from build123d import *

# Parameters (mm, degrees)
SKETCH1_R                    = 203.2
BOSS_EXTRUDE1_DEPTH          = 6.35
F_0_257_DIAMETER_HOLE1_D     = 6.5278
CIRPATTERN1_COUNT            = 36
F_1_2_0_5_DIAMETER_HOLE1_D   = 12.7
F_3_8_0_375_DIAMETER_HOLE1_D = 9.525
CIRPATTERN2_COUNT            = 4
F_3_8_0_375_DIAMETER_HOLE2_D = 9.525
LPATTERN1_COUNT              = 2
LPATTERN1_PITCH              = 254
LPATTERN1_COUNT_DIR2         = 2
LPATTERN1_PITCH_DIR2         = 76.2


with BuildPart() as part:
    # Sketch1 → Boss-Extrude1 (new body)
    with BuildSketch(Plane(origin=(0, 0, 0), x_dir=(0, 0, -1), z_dir=(1, 0, 0))):
        Circle(SKETCH1_R)
    extrude(amount=BOSS_EXTRUDE1_DEPTH)

    # F (0.257) Diameter Hole1 (through all)
    with Locations(Plane(origin=(6.35, 0, 0), x_dir=(0, 0, -1), z_dir=(1, 0, 0))):
        with Locations((-196.85, 0)):
            f_0_257_diameter_hole1 = Hole(F_0_257_DIAMETER_HOLE1_D / 2)

    # CirPattern1: F (0.257) Diameter Hole1 ×36 about axis
    cirpattern1_axis = Axis((0, 0, 0), (-1, 0, 0))
    for i in range(1, CIRPATTERN1_COUNT):
        add(f_0_257_diameter_hole1.rotate(cirpattern1_axis, i * 360 / CIRPATTERN1_COUNT), mode=Mode.SUBTRACT)

    # 1/2 (0.5) Diameter Hole1 (through all)
    with Locations(Plane(origin=(6.35, 0, 0), x_dir=(0, 0, -1), z_dir=(1, 0, 0))):
        with Locations((0, 0)):
            Hole(F_1_2_0_5_DIAMETER_HOLE1_D / 2)

    # 3/8 (0.375) Diameter Hole1 (through all)
    with Locations(Plane(origin=(6.35, 0, 0), x_dir=(0, 0, -1), z_dir=(1, 0, 0))):
        with Locations((0, -76.2)):
            f_3_8_0_375_diameter_hole1 = Hole(F_3_8_0_375_DIAMETER_HOLE1_D / 2)

    # CirPattern2: 3/8 (0.375) Diameter Hole1 ×4 about axis
    cirpattern2_axis = Axis((0, 0, 0), (-1, 0, 0))
    for i in range(1, CIRPATTERN2_COUNT):
        add(f_3_8_0_375_diameter_hole1.rotate(cirpattern2_axis, i * 360 / CIRPATTERN2_COUNT), mode=Mode.SUBTRACT)

    # 3/8 (0.375) Diameter Hole2 (through all)
    with Locations(Plane(origin=(6.35, 0, 0), x_dir=(0, 0, -1), z_dir=(1, 0, 0))):
        with Locations((-127, -38.1)):
            f_3_8_0_375_diameter_hole2 = Hole(F_3_8_0_375_DIAMETER_HOLE2_D / 2)

    # LPattern1: 3_8 _0.375_ Diameter Hole2 2 × 2
    with Locations(*[(0, j * LPATTERN1_PITCH_DIR2, -i * LPATTERN1_PITCH) for i in range(LPATTERN1_COUNT) for j in range(LPATTERN1_COUNT_DIR2) if (i, j) != (0, 0)]):
        add(f_3_8_0_375_diameter_hole2, mode=Mode.SUBTRACT)


solid = part.part
Work out the finished part from the listing and answer in its coordinate system (mm). Give positions to 0.01 mm unless a question says otherwise; leave off trailing zeros. Loops run counter-clockwise (first coordinate to the right, second up) from the corner with the lowest first, then second, coordinate; pieces in that order, holes last. Notation, with made-up numbers: (-8, -6) - (24, -6) arc R19 cw to (24, 24) - close; hole circle Ø10 at (-28.5, 38). An arc over 180 degrees is marked (long way). Answer in a Markdown table with one row per item.
(1) A flat-ended cylindrical pin translates along its axis: pin 1 Ø4 at (y, z) = (-170.48, -98.43) entering from -X. Find the tip coordinate at first contact, or state that the pin passes through.
Results list:
| item | result |
|---|---|
| pin 1 | passes through |
(2) Consider L1, parallel to Y at x = 4.5, z = -66; L2, parallel to Z at x = 3.5, y = 67.5; L3, parallel to Y at x = 2.5, z = -1.5. Determine where each line is inside the solid, lowest interval first. Write a range as [from, to].
Results list:
| item | result |
|---|---|
| L1 | y = [-192.18, -187.96], [-182, 182], [187.96, 192.18] |
| L2 | z = [-191.66, -188.24], [-181.72, 181.72], [188.24, 191.66] |
| L3 | y = [-203.19, -199.75], [-193.95, -80.72], [-71.68, -6.17], [6.17, 71.68], [80.72, 193.95], [199.75, 203.19] |
(3) Section D-D (y = -54.5) is taken. Give the vertices of the cut face in (x, z), and give its area (3 significant figures).
Results list:
| item | result |
|---|---|
| outline | (0, -195.75) - (6.35, -195.75) - (6.35, 195.75) - (0, 195.75) - close |
| area | 2,490 mm² |
(4) Section A-A (y = 76.2) is taken. Give the vertices of the cut face in (x, z), and give its area (3 significant figures).
Results list:
| item | result |
|---|---|
| outline | (0, -188.37) - (6.35, -188.37) - (6.35, -4.76) - (0, -4.76) - close; (0, 4.76) - (6.35, 4.76) - (6.35, 188.37) - (0, 188.37) - close |
| area | 2,330 mm² |
(5) For a pull along Z with two mould halves and no side action, classify faces 1 (the face through (3.13, -41, 123.22)), 2 (the face through (3.131, -198.368, 44.05)), 3 (the face through (6.35, 3, -42)), 4 (the face through (3.13, 71.48, 0.62)) as pulls with the +Z half, pulls with the -Z half, needs draft (parallel to the pull), parting line crosses it, or undercut.
Results list:
| item | result |
|---|---|
| face 1 | undercut |
| face 2 | parting line crosses it |
| face 3 | needs draft |
| face 4 | undercut |
(6) Section B-B (x = 1.25) is taken. State how many separate pieces and enclosed holes the cut face has, and give its area (3 significant figures).
Results list:
| item | result |
|---|---|
| separate pieces | 1 |
| enclosed holes | 45 |
| area | 128,000 mm² |
(7) Section C-C (y = -136) is taken. Give the vertices of the cut face in (x, z), and give its area (3 significant figures).
Results list:
| item | result |
|---|---|
| outline | (0, -150.98) - (6.35, -150.98) - (6.35, 150.98) - (0, 150.98) - close |
| area | 1,920 mm² |
